Part model, mm, in its own coordinate system. A direction names the side the tool comes from. Round coordinates to 2 decimals unless told otherwise and drop trailing zeros. Write each loop counter-clockwise with the first axis right and the second up, starting at its lowest first coordinate (ties: lowest second). Pieces come first, ordered by that corner, then holes. Notation, with made-up numbers: (6.5, -1.75) -> (46.5, -1.75) arc R30 cw to (46.5, 35.25) -> close; hole circle Ø6 at (19.25, 85.25). An arc over 180 degrees is marked (long way). Return JSON: item names as keys, results as strings. Group by question number.
```python
from build123d import *

# Parameters (mm, degrees)
SALIENTE_EXTRUIR1_DEPTH          = 35
SALIENTE_EXTRUIR2_DEPTH          = 35
CROQUIS3_W                       = 180
CROQUIS3_H                       = 65
SALIENTE_EXTRUIR3_DEPTH          = 3
REDONDEO1_R                      = 20
CROQUIS5_R                       = 2.5
CROQUIS5_R_2                     = 2.75
CORTAR_EXTRUIR1_DEPTH            = 3
CORTAR_EXTRUIR3_REACH            = 103.888
CROQUIS7_R                       = 1.75
TALADRO_DE_MARGEN_PARA_M31_D     = 3.4
TALADRO_DE_MARGEN_PARA_M31_DEPTH = 30
TALADRO_DE_MARGEN_PARA_M31_TIP   = 1.021463052
CORTAR_EXTRUIR4_REACH            = 104.958
CROQUIS10_R                      = 1.75
CROQUIS11_R                      = 5
CORTAR_EXTRUIR5_DEPTH            = 10
CROQUIS12_R                      = 6.5
CORTAR_EXTRUIR6_DEPTH            = 10
CROQUIS13_R                      = 11
CROQUIS13_R_2                    = 8.15
SALIENTE_EXTRUIR4_DEPTH          = 7
REDONDEO2_R                      = 5


with BuildPart() as part:
    # Croquis1 → Saliente-Extruir1 (new body)
    with BuildSketch(Plane(origin=(0, 0, 0), x_dir=(1, 0, 0), z_dir=(0, 1, 0))):
        Polygon((90, -32.5), (90, 0), (87, 0), (87, -29.5), (-87, -29.5), (-87, 0), (-90, 0), (-90, -32.5), align=None)
        Polygon((87, 0), (90, 0), (90, 32.5), (-90, 32.5), (-90, 0), (-87, 0), (-87, 29.5), (87, 29.5), align=None)
    extrude(amount=SALIENTE_EXTRUIR1_DEPTH)

    # Croquis2 → Saliente-Extruir2 (add)
    with BuildSketch(Plane(origin=(0, 35, 0), x_dir=(1, 0, 0), z_dir=(0, 1, 0))):
        Polygon((87, 29.5), (67, 29.5), (87, 9.5), align=None)
        Polygon((-67, 29.5), (-87, 9.5), (-87, 29.5), align=None)
        Polygon((67, -29.5), (87, -9.5), (87, -29.5), align=None)
        Polygon((-87, -29.5), (-67, -29.5), (-87, -9.5), align=None)
    extrude(amount=-SALIENTE_EXTRUIR2_DEPTH)

    # Croquis3 → Saliente-Extruir3 (add)
    with BuildSketch(Plane(origin=(0, 35, 0), x_dir=(1, 0, 0), z_dir=(0, 1, 0))):
        Rectangle(CROQUIS3_W, CROQUIS3_H)
    extrude(amount=SALIENTE_EXTRUIR3_DEPTH)

    # Redondeo1
    redondeo1_edges = [part.edges().sort_by_distance(p)[0] for p in [
        (90, 19, -32.5),
        (90, 19, 32.5),
        (-90, 19, 32.5),
        (-90, 19, -32.5),
    ]]
    fillet(redondeo1_edges, radius=REDONDEO1_R)

    # Croquis5 → Cortar-Extruir1 (cut)
    with BuildSketch(Plane.XZ.offset(-35)):
        with Locations(Location((-67, 0, 0), (0, 0, 270))):
            Circle(CROQUIS5_R)
        with Locations(Location((-25, 0, 0), (0, 0, 270))):
            Circle(CROQUIS5_R_2)
        with Locations(Location((45, 0, 0), (0, 0, 270))):
            Circle(CROQUIS5_R_2)
    extrude(amount=-CORTAR_EXTRUIR1_DEPTH, mode=Mode.SUBTRACT)

    # Croquis7 → Cortar-Extruir3 (cut, up to next)
    with BuildSketch(Plane.XZ.offset(-35), mode=Mode.PRIVATE) as cortar_extruir3_sk1:
        with Locations(Location((-67, 16, 0), (0, 0, 270))):
            Circle(CROQUIS7_R)
    cortar_extruir3_tool1 = extrude(cortar_extruir3_sk1.sketch, amount=-CORTAR_EXTRUIR3_REACH, mode=Mode.PRIVATE) & part.part
    # Croquis7 → Cortar-Extruir3 (cut, up to next)
    with BuildSketch(Plane.XZ.offset(-35), mode=Mode.PRIVATE) as cortar_extruir3_sk2:
        with Locations(Location((-59, 0, 0), (0, 0, 270))):
            Circle(CROQUIS7_R)
    cortar_extruir3_tool2 = extrude(cortar_extruir3_sk2.sketch, amount=-CORTAR_EXTRUIR3_REACH, mode=Mode.PRIVATE) & part.part
    # Croquis7 → Cortar-Extruir3 (cut, up to next)
    with BuildSketch(Plane.XZ.offset(-35), mode=Mode.PRIVATE) as cortar_extruir3_sk3:
        with Locations(Location((-67, -16, 0), (0, 0, 270))):
            Circle(CROQUIS7_R)
    cortar_extruir3_tool3 = extrude(cortar_extruir3_sk3.sketch, amount=-CORTAR_EXTRUIR3_REACH, mode=Mode.PRIVATE) & part.part
    # Croquis7 → Cortar-Extruir3 (cut, up to next)
    with BuildSketch(Plane.XZ.offset(-35), mode=Mode.PRIVATE) as cortar_extruir3_sk4:
        with Locations(Location((-75, 0, 0), (0, 0, 270))):
            Circle(CROQUIS7_R)
    cortar_extruir3_tool4 = extrude(cortar_extruir3_sk4.sketch, amount=-CORTAR_EXTRUIR3_REACH, mode=Mode.PRIVATE) & part.part
    add(cortar_extruir3_tool1.solids().sort_by_distance((-67, 35, 16))[0], mode=Mode.SUBTRACT)
    add(cortar_extruir3_tool2.solids().sort_by_distance((-59, 35, 0))[0], mode=Mode.SUBTRACT)
    add(cortar_extruir3_tool3.solids().sort_by_distance((-67, 35, -16))[0], mode=Mode.SUBTRACT)
    add(cortar_extruir3_tool4.solids().sort_by_distance((-75, 35, 0))[0], mode=Mode.SUBTRACT)

    # Taladro de margen para M31
    with Locations(Plane.XZ):
        with Locations((-80, 22.5), (80, 22.5), (-80, -22.5), (80, -22.5)):
            Hole(TALADRO_DE_MARGEN_PARA_M31_D / 2, depth=TALADRO_DE_MARGEN_PARA_M31_DEPTH)
            with Locations((0, 0, -(TALADRO_DE_MARGEN_PARA_M31_DEPTH + TALADRO_DE_MARGEN_PARA_M31_TIP / 2))):  # 118° drill point
                Cone(0, TALADRO_DE_MARGEN_PARA_M31_D / 2, TALADRO_DE_MARGEN_PARA_M31_TIP, mode=Mode.SUBTRACT)

    # Croquis10 → Cortar-Extruir4 (cut, up to next)
    with BuildSketch(Plane(origin=(0, 38, 0), x_dir=(1, 0, 0), z_dir=(0, 1, 0)), mode=Mode.PRIVATE) as cortar_extruir4_sk1:
        with Locations(Location((-25, 8.5, 0), (0, 0, 270))):
            Circle(CROQUIS10_R)
    cortar_extruir4_tool1 = extrude(cortar_extruir4_sk1.sketch, amount=-CORTAR_EXTRUIR4_REACH, mode=Mode.PRIVATE) & part.part
    # Croquis10 → Cortar-Extruir4 (cut, up to next)
    with BuildSketch(Plane(origin=(0, 38, 0), x_dir=(1, 0, 0), z_dir=(0, 1, 0)), mode=Mode.PRIVATE) as cortar_extruir4_sk2:
        with Locations(Location((-16.5, 0, 0), (0, 0, 270))):
            Circle(CROQUIS10_R)
    cortar_extruir4_tool2 = extrude(cortar_extruir4_sk2.sketch, amount=-CORTAR_EXTRUIR4_REACH, mode=Mode.PRIVATE) & part.part
    # Croquis10 → Cortar-Extruir4 (cut, up to next)
    with BuildSketch(Plane(origin=(0, 38, 0), x_dir=(1, 0, 0), z_dir=(0, 1, 0)), mode=Mode.PRIVATE) as cortar_extruir4_sk3:
        with Locations(Location((-25, -8.5, 0), (0, 0, 270))):
            Circle(CROQUIS10_R)
    cortar_extruir4_tool3 = extrude(cortar_extruir4_sk3.sketch, amount=-CORTAR_EXTRUIR4_REACH, mode=Mode.PRIVATE) & part.part
    # Croquis10 → Cortar-Extruir4 (cut, up to next)
    with BuildSketch(Plane(origin=(0, 38, 0), x_dir=(1, 0, 0), z_dir=(0, 1, 0)), mode=Mode.PRIVATE) as cortar_extruir4_sk4:
        with Locations(Location((-33.5, 0, 0), (0, 0, 270))):
            Circle(CROQUIS10_R)
    cortar_extruir4_tool4 = extrude(cortar_extruir4_sk4.sketch, amount=-CORTAR_EXTRUIR4_REACH, mode=Mode.PRIVATE) & part.part
    add(cortar_extruir4_tool1.solids().sort_by_distance((-25, 38, -8.5))[0], mode=Mode.SUBTRACT)
    add(cortar_extruir4_tool2.solids().sort_by_distance((-16.5, 38, 0))[0], mode=Mode.SUBTRACT)
    add(cortar_extruir4_tool3.solids().sort_by_distance((-25, 38, 8.5))[0], mode=Mode.SUBTRACT)
    add(cortar_extruir4_tool4.solids().sort_by_distance((-33.5, 38, 0))[0], mode=Mode.SUBTRACT)

    # Croquis11 → Cortar-Extruir5 (cut)
    with BuildSketch(Plane.XZ.offset(-35)):
        with Locations(Location((-35, -17.5, 0), (0, 0, 270))):
            Circle(CROQUIS11_R)
    extrude(amount=-CORTAR_EXTRUIR5_DEPTH, mode=Mode.SUBTRACT)

    # Croquis12 → Cortar-Extruir6 (cut)
    with BuildSketch(Plane(origin=(0, 38, 0), x_dir=(1, 0, 0), z_dir=(0, 1, 0))):
        with Locations(Location((45, 0, 0), (0, 0, 270))):
            Circle(CROQUIS12_R)
    extrude(amount=-CORTAR_EXTRUIR6_DEPTH, mode=Mode.SUBTRACT)

    # Croquis13 → Saliente-Extruir4 (add)
    with BuildSketch(Plane(origin=(0, 38, 0), x_dir=(1, 0, 0), z_dir=(0, 1, 0))):
        with Locations(Location((45, 0, 0), (0, 0, 90))):
            Circle(CROQUIS13_R)
        with Locations(Location((45, 0, 0), (0, 0, 270))):
            Circle(CROQUIS13_R_2, mode=Mode.SUBTRACT)
    extrude(amount=SALIENTE_EXTRUIR4_DEPTH)

    # Redondeo2
    redondeo2_edges = [part.edges().sort_by_distance(p)[0] for p in [
        (45, 38, 11),
    ]]
    fillet(redondeo2_edges, radius=REDONDEO2_R)


solid = part.part
```
Item 1: Cut at D-D (z = 0). State how many separate pieces and enclosed holes the cut face has, then the cut area to 3 significant figures.
Item 2: Cut at A-A (x = -25). Write the cut outline in (y, z), then the cut area to 4 significant figures.
Item 3: Two-plate mould, pull along Z, no slides. Class faces 1 (the face through (84.297, 18.734, -26.486)), 2 (the face through (-87, 17, 0)), 3 (the face through (-84.297, 19.266, 26.486)): released by +Z, released by -Z, zero draft, split by the parting line, or undercut.
Item 4: Which spindle directions (+Z, -Z, +X, -X, +Y, -Y) get a long thin tool onto all of the face, cutting with end or side? Do faces 4 (the face through (53.08, 41.45, -1.06)), 5 (the face through (-68.71, 36.48, -15.62)), 6 (the face through (87, 17, 0)). Say none if no direction does.
Item 5: Wall check: L1, parallel to X at y = 13.5, z = 0; L2, parallel to Z at x = -80, y = 15; L3, parallel to Z at x = 47, y = 5. Give the ranges that are in metal, low to high.
Item 6: Cut at C-C (x = -59). Write the cut outline in (y, z).
Item 7: Flat gauge pins, fed straight in: P1, Ø6, axis at x = -54, z = -10, coming from the +Y side; P2, Ø4, axis at x = -25, z = 8.5, coming from the -Y side; P3, Ø11.5, axis at x = 45, z = 0, coming from the -Y side; P4, Ø3, axis at x = -80, z = -22.5, coming from the -Y side. Where does each tip first touch, or does it go through?
Item 8: Cut at B-B (y = 14.5). Write the cut outline in (x, z), then the cut area to 3 significant figures.
Checks:
{
 "1": {"separate pieces": "8", "enclosed holes": "0", "area": "688 mm2"},
 "2": {"outline": "(0, -32.5) -> (38, -32.5) -> (38, -10.25) -> (35, -10.25) -> (35, -29.5) -> (0, -29.5) -> close; (0, 29.5) -> (35, 29.5) -> (35, 10.25) -> (38, 10.25) -> (38, 32.5) -> (0, 32.5) -> close; (35, -6.75) -> (38, -6.75) -> (38, -2.75) -> (35, -2.75) -> close; (35, 2.75) -> (38, 2.75) -> (38, 6.75) -> (35, 6.75) -> close", "area": "367.5 mm2"},
 "3": {"face 1": "released by -Z", "face 2": "undercut", "face 3": "released by +Z"},
 "4": {"face 4": "+Y", "face 5": "+Y, -Y", "face 6": "-Y"},
 "5": {"L1": "x = -90 to -87, 87 to 90", "L2": "z = -29.82 to -24.2, -20.8 to -16.5, 16.5 to 20.8, 24.2 to 29.82", "L3": "z = -32.5 to -29.5, 29.5 to 32.5"},
 "6": {"outline": "(0, -32.5) -> (38, -32.5) -> (38, -1.75) -> (35, -1.75) -> (35, -29.5) -> (0, -29.5) -> close; (0, 29.5) -> (35, 29.5) -> (35, 1.75) -> (38, 1.75) -> (38, 32.5) -> (0, 32.5) -> close"},
 "7": {"P1": "stops at y = 38", "P2": "stops at y = 35", "P3": "passes through", "P4": "stops at y = 30.12"},
 "8": {"outline": "(-90, -12.5) arc R20 ccw to (-70, -32.5) -> (70, -32.5) arc R20 ccw to (90, -12.5) -> (90, 12.5) arc R20 ccw to (70, 32.5) -> (-70, 32.5) arc R20 ccw to (-90, 12.5) -> close; hole (-87, -9.5) -> (-67, -29.5) -> (67, -29.5) -> (87, -9.5) -> (87, 9.5) -> (67, 29.5) -> (-67, 29.5) -> (-87, 9.5) -> close; hole circle Ø3.4 at (-80, -22.5); hole circle Ø3.4 at (-80, 22.5); hole circle Ø3.4 at (80, -22.5); hole circle Ø3.4 at (80, 22.5)", "area": "1,850 mm2"}
}
